Design review of the part built by this model. Coordinates are the model's own, in mm. Face numbers are marked on the shaded views. A direction names the side the tool comes from. Round coordinates to 2 decimals unless told otherwise and drop trailing zeros. Write each loop counter-clockwise with the first axis right and the second up, starting at its lowest first coordinate (ties: lowest second). Pieces come first, ordered by that corner, then holes.
from build123d import *

# Parameters (mm, degrees)
SKETCH1_W           = 175
SKETCH1_H           = 90
BOSS_EXTRUDE1_DEPTH = 80
SKETCH2_W           = 155
SKETCH2_H           = 60
CUT_EXTRUDE1_DEPTH  = 80
SKETCH3_W           = 60
SKETCH3_H           = 60
CUT_EXTRUDE2_DEPTH  = 176
SKETCH4_R           = 52.5
BOSS_EXTRUDE3_DEPTH = 20
CUT_EXTRUDE3_DEPTH  = 20
SKETCH6_R           = 4.715207805
CUT_EXTRUDE4_DEPTH  = 20
CIRPATTERN1_COUNT   = 7
SKETCH7_R           = 15
CUT_EXTRUDE5_DEPTH  = 20


with BuildPart() as part:
    # Sketch1 → Boss-Extrude1 (new body)
    with BuildSketch(Plane(origin=(0, 0, 0), x_dir=(1, 0, 0), z_dir=(0, 1, 0))):
        Rectangle(SKETCH1_W, SKETCH1_H)
    extrude(amount=BOSS_EXTRUDE1_DEPTH)

    # Sketch2 → Cut-Extrude1 (cut)
    with BuildSketch(Plane(origin=(0, 80, 0), x_dir=(1, 0, 0), z_dir=(0, 1, 0))):
        with Locations((0, 5)):
            Rectangle(SKETCH2_W, SKETCH2_H)
    extrude(amount=-CUT_EXTRUDE1_DEPTH, mode=Mode.SUBTRACT)

    # Sketch3 → Cut-Extrude2 (cut, through all)
    with BuildSketch(Plane(origin=(87.5, 0, 0), x_dir=(0, 0, -1), z_dir=(1, 0, 0))):
        with Locations((5, 40)):
            Rectangle(SKETCH3_W, SKETCH3_H)
    extrude(amount=-CUT_EXTRUDE2_DEPTH, mode=Mode.SUBTRACT)

    # Sketch4 → Boss-Extrude3 (add)
    with BuildSketch(Plane.XY.offset(45)):
        with Locations((0, 40)):
            Circle(SKETCH4_R)
    extrude(amount=-BOSS_EXTRUDE3_DEPTH)

    # Sketch5 → Cut-Extrude3 (cut)
    with BuildSketch(Plane.XY.offset(45)):
        with BuildLine():
            Line((87.5, 70), (43.084219849, 70))
            ThreePointArc((43.084219849, 70), (52.5, 40), (43.084219849, 10))
            Line((43.084219849, 10), (87.5, 10))
            Line((87.5, 10), (87.5, 70))
        make_face()
        with BuildLine():
            Line((-43.084219849, 70), (-87.5, 70))
            Line((-87.5, 70), (-87.5, 10))
            Line((-87.5, 10), (-43.084219849, 10))
            ThreePointArc((-43.084219849, 10), (-52.5, 40), (-43.084219849, 70))
        make_face()
    extrude(amount=-CUT_EXTRUDE3_DEPTH, mode=Mode.SUBTRACT)

    # Sketch6 → Cut-Extrude4 (cut)
    with BuildSketch(Plane.XY.offset(45)):
        with Locations((40, 40)):
            Circle(SKETCH6_R)
    cut_extrude4 = extrude(amount=-CUT_EXTRUDE4_DEPTH, mode=Mode.SUBTRACT)

    # CirPattern1: Cut-Extrude4 ×7 about axis
    cirpattern1_axis = Axis((0, 40, 0), (0, 0, 1))
    for i in range(1, CIRPATTERN1_COUNT):
        add(cut_extrude4.rotate(cirpattern1_axis, i * 360 / CIRPATTERN1_COUNT), mode=Mode.SUBTRACT)

    # Sketch7 → Cut-Extrude5 (cut)
    with BuildSketch(Plane.XY.offset(45)):
        with Locations((0, 40)):
            Circle(SKETCH7_R)
    extrude(amount=-CUT_EXTRUDE5_DEPTH, mode=Mode.SUBTRACT)


solid = part.part
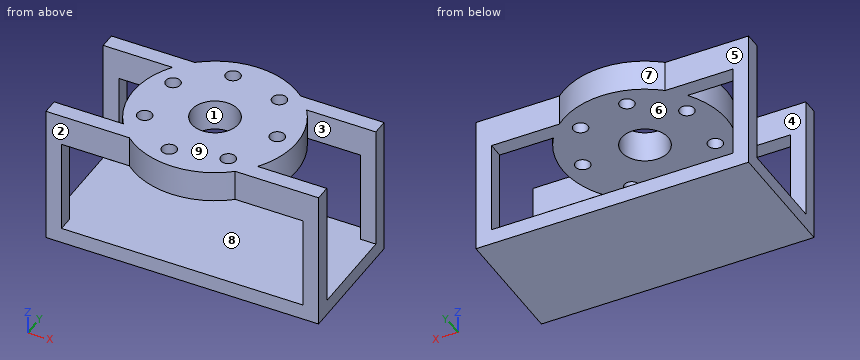
1) Add section D-D on x = 66. State the section outline as (y, z) points.
2) For the marked faces 1, 2, 3, 4 and 5, list the 3-axis set-ups (+Z, -Z, +X, -X, +Y, -Y) from which the entire face can be reached by the end or side of a thin tool; tool diameter is ignored.
3) The part is to be moulded in two halves that separate along Z. For the marked faces 6, 7, 8 and 9, say which applies: pulls with the +Z half, pulls with the -Z half, needs draft (parallel to the pull), parting line crosses it, or undercut.
4) For P1, Ø6, axis at x = 69.5, y = 11, coming from the +Z side; P2, Ø1, axis at x = -61, z = 25, coming from the -Y side; P3, Ø1.5, axis at y = 63, z = 28.5, coming from the +X side; P4, Ø8.5, axis at x = -36.04, y = 57.36, coming from the +Z side, all flat-tipped, find the tip position at first contact; note any pin that passes through.
5) For line 1 along X through (y, z) = (78.5, 5.5); line 2 along Z through (x, y) = (2, 10); line 3 along Y through (x, z) = (40, 34.25), list the stretches that pass through material, from the lowest coordinate up.
6) Add section C-C on z = -3. State the section outline as (x, y) points, and give its area (3 significant figures).
7) Add section A-A on x = 0. State the section outline as (y, z) points.
8) Add section B-B on y = 40. State the section outline as (x, z) points.
Computed:
1. outline: (0, -45) - (80, -45) - (80, -35) - (0, -35) - close; (0, 25) - (10, 25) - (10, 45) - (0, 45) - close; (70, 25) - (80, 25) - (80, 45) - (70, 45) - close
2. face 1: +Z
2. face 2: -Z, -Y
2. face 3: +Z, +X
2. face 4: +Z, -X
2. face 5: -Z, +Y
3. face 6: undercut
3. face 7: needs draft
3. face 8: undercut
3. face 9: pulls with the +Z half
4. P1: stops at z = 45
4. P2: stops at y = 0
4. P3: stops at x = 47.55
4. P4: stops at z = -35
5. line 1: x = -87.5 to -77.5, 77.5 to 87.5
5. line 2: z = -45 to -35, 25 to 45
5. line 3: y = 0 to 35.28, 44.72 to 80
6. outline: (-87.5, 0) - (-77.5, 0) - (-77.5, 10) - (-87.5, 10) - close; (-87.5, 70) - (-77.5, 70) - (-77.5, 80) - (-87.5, 80) - close; (77.5, 0) - (87.5, 0) - (87.5, 10) - (77.5, 10) - close; (77.5, 70) - (87.5, 70) - (87.5, 80) - (77.5, 80) - close
6. area: 400 mm2
7. outline: (-12.5, 25) - (25, 25) - (25, 45) - (-12.5, 45) - close; (0, -45) - (80, -45) - (80, -35) - (0, -35) - close; (55, 25) - (92.5, 25) - (92.5, 45) - (55, 45) - close
8. outline: (-87.5, -45) - (87.5, -45) - (87.5, -35) - (-87.5, -35) - close; (-52.5, 25) - (-15, 25) - (-15, 45) - (-52.5, 45) - close; (15, 25) - (35.28, 25) - (35.28, 45) - (15, 45) - close; (44.72, 25) - (52.5, 25) - (52.5, 45) - (44.72, 45) - close
